Part print with two shaded views. Sizes in mm from the minimum x, y, z corner. Round coordinates to 2 decimals unless told otherwise and drop trailing zeros. Write each loop counter-clockwise with the first axis right and the second up, starting at its lowest first coordinate (ties: lowest second). Pieces come first, ordered by that corner, then holes. Notation, with made-up numbers: M 48.25,50 L 95.25,50 A10 cw 95.25,65 Z; hole C 66.25,23 d11. An arc over 180 degrees is marked long. One line per question, with ' | ' between items. Start each with the question number.
1) Wall check: probe 1 along Z at (x, y) = (33, 8.75); probe 2 along X at (y, z) = (11, 40); probe 3 along X at (y, z) = (18.25, 59.5) (1 decimal). Give the ranges that are in metal, low to high. Write a range as [from, to].
2) Mould opens along Z. For the marked faces 1, 2 and 3 say: pulls with the +Z half, pulls with the -Z half, needs draft (parallel to the pull), parting line crosses it, or undercut.
3) Saw through at A-A (z = 31). Give the number of separate pieces and of enclosed holes in the cut face, plus the area to 4 significant figures.
4) Drop flat-ended pins along their axis: pin 1 Ø3 at (y, z) = (15, 25) entering from +X; pin 2 Ø4 at (x, y) = (20.5, 20.5) entering from -Z; pin 3 Ø5 at (y, z) = (12.5, 30) entering from -X. Give the stop position or say it passes through.
5) Saw through at D-D (z = 52). List the corners of the cut face in (x, y).
6) Saw through at B-B (x = 49). List the corners of the cut face in (y, z).
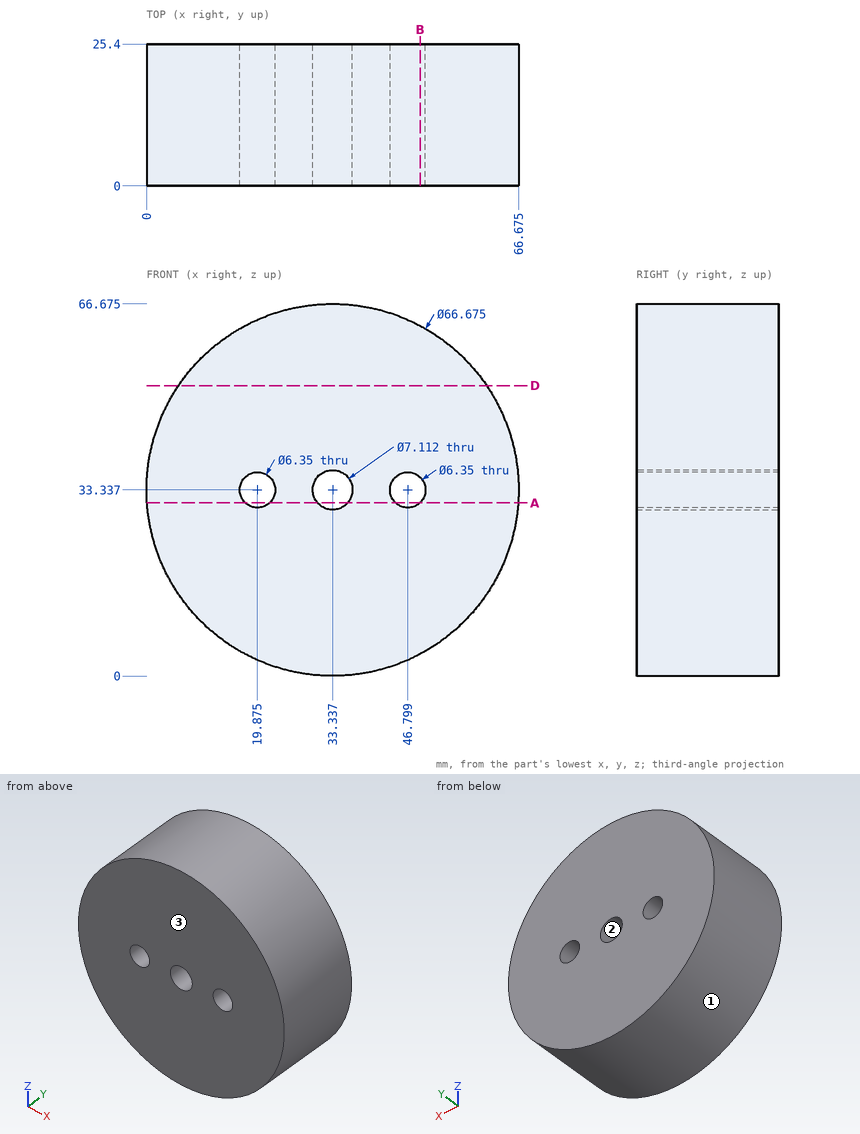
Answer key:
1) probe 1: z = [0, 29.8], [36.88, 66.67] | probe 2: x = [0.67, 66] | probe 3: x = [12.7, 54]
2) face 1: parting line crosses it | face 2: undercut | face 3: needs draft
3) separate pieces: 4 | enclosed holes: 0 | area: 1,335 mm2
4) pin 1: stops at x = 65.97 | pin 2: stops at z = 1.81 | pin 3: stops at x = 0.01
5) outline: M 5.71,0 L 60.96,0 L 60.96,25.4 L 5.71,25.4 Z
6) outline: M 0,3.91 L 25.4,3.91 L 25.4,31.05 L 0,31.05 Z; M 0,35.63 L 25.4,35.63 L 25.4,62.77 L 0,62.77 Z
